The listing builds one solid part. Answer for the finished solid, in the listing's coordinates (mm). Give positions to 0.01 mm unless a question says otherwise; leave off trailing zeros. Write each loop counter-clockwise with the first axis right and the second up, starting at its lowest first coordinate (ties: lowest second). Pieces come first, ordered by that corner, then holes. Notation, with made-up numbers: M -10,25.5 L 18,25.5 A29 cw 18,58.5 Z; hole C -31,-17 d1. An arc over 180 degrees is marked long. Return JSON: item names as keys, results as strings.
from build123d import *

# Parameters (mm, degrees)
F2_DEPTH = 28.4
F3_DEPTH = 4
F6_D     = 5
F6_DEPTH = 5
F6_TIP   = 1.5021515476
F7_D     = 5
F7_DEPTH = 7
F7_TIP   = 1.5021515476
F8_R     = 1
F9_R     = 1.4485281374


with BuildPart() as f2:
    # F0 (on Front) → F2 (new body)
    with BuildSketch(Plane.XZ):
        with BuildLine():
            Line((23.6029717884, 8.2401288069), (37.7647548615, 13.1842060911))
            ThreePointArc((37.7647548615, 13.1842060911), (30.9779974122, 25.3054080451), (20.4548362885, 34.3744043208))
            Line((20.4548362885, 34.3744043208), (12.7842726803, 21.4840027005))
            ThreePointArc((12.7842726803, 21.4840027005), (19.3612483826, 15.8158800282), (23.6029717884, 8.2401288069))
        make_face()
    extrude(amount=F2_DEPTH)

    # F1 (on Front) + F0 (on Front) → F3 (join)
    with BuildSketch(Plane.XZ):
        with BuildLine():
            ThreePointArc((15.2340019476, 15.8721512297), (17.0378985767, 13.9179744248), (18.5928148308, 11.7604097152))
            Line((18.5928148308, 11.7604097152), (21.4911474241, 12.7722583124))
            ThreePointArc((21.4911474241, 12.7722583124), (22.6606475272, 10.5591218219), (23.6029717884, 8.2401288069))
            Line((23.6029717884, 8.2401288069), (37.7647548615, 13.1842060911))
            ThreePointArc((37.7647548615, 13.1842060911), (30.9779974122, 25.3054080451), (20.4548362885, 34.3744043208))
            Line((20.4548362885, 34.3744043208), (12.7842726803, 21.4840027005))
            ThreePointArc((12.7842726803, 21.4840027005), (14.8685909795, 20.0978855177), (16.8038497839, 18.5102845046))
            Line((16.8038497839, 18.5102845046), (15.2340019476, 15.8721512297))
        make_face()
    with BuildSketch(Plane.XZ):
        with BuildLine():
            Line((23.6029717884, 8.2401288069), (37.7647548615, 13.1842060911))
            ThreePointArc((37.7647548615, 13.1842060911), (30.9779974122, 25.3054080451), (20.4548362885, 34.3744043208))
            Line((20.4548362885, 34.3744043208), (12.7842726803, 21.4840027005))
            ThreePointArc((12.7842726803, 21.4840027005), (19.3612483826, 15.8158800282), (23.6029717884, 8.2401288069))
        make_face()
    extrude(amount=-F3_DEPTH)

    # F6 (one way)
    with BuildSketch(Plane(origin=(29.109795575, 0, 23.7793052059), x_dir=(0, 1, 0), z_dir=(-0.7744499353, 0, -0.6326352011))):
        with Locations((-5, 0)):
            Circle(F6_D / 2)
    extrude(amount=-F6_DEPTH, mode=Mode.SUBTRACT)
    with Locations(Plane(origin=(29.109795575, 0, 23.7793052059), x_dir=(0, 1, 0), z_dir=(-0.7744499353, 0, -0.6326352011))):
        with Locations((-5, 0)):
            with Locations((0, 0, -(F6_DEPTH + F6_TIP / 2))):  # 118° drill point
                Cone(0, F6_D / 2, F6_TIP, mode=Mode.SUBTRACT)

    # F7
    with Locations(Plane(origin=(29.109795575, 0, 23.7793052059), x_dir=(0, 1, 0), z_dir=(0.7744499353, 0, 0.6326352011))):
        with Locations((-5, 0)):
            Hole(F7_D / 2, depth=F7_DEPTH)
            with Locations((0, 0, -(F7_DEPTH + F7_TIP / 2))):  # 118° drill point
                Cone(0, F7_D / 2, F7_TIP, mode=Mode.SUBTRACT)

    # F8
    f8_edges = [f2.edges().sort_by_distance(p)[0] for p in [
        (21.491147, 2, 12.772258),
        (16.80385, 2, 18.510285),
    ]]
    fillet(f8_edges, radius=F8_R)

    # F9
    f9_edges = [f2.edges().sort_by_distance(p)[0] for p in [
        (17.037899, 4, 13.917974),
        (16.505655, 4, 18.471804),
        (21.393938, 4, 12.487739),
    ]]
    fillet(f9_edges, radius=F9_R)


solid = f2.part
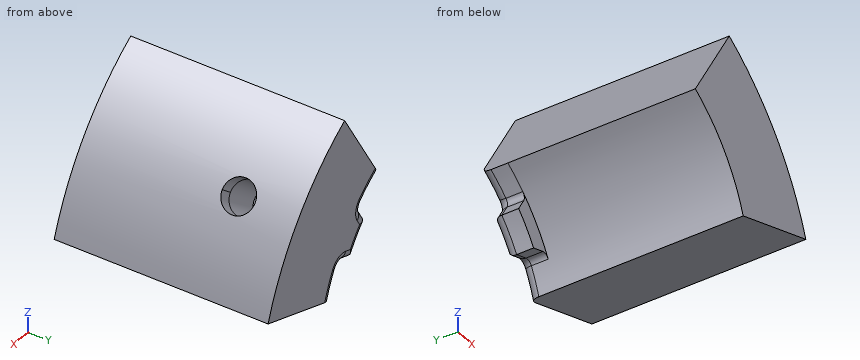
Item 1: Given pin 1 Ø8 at (y, z) = (-23.5, 27.5) entering from -X; pin 2 Ø6 at (x, y) = (34, -16.5) entering from -Z; pin 3 Ø10 at (y, z) = (-12, 15.5) entering from +X, each flat-ended and moving along its own axis, determine where each tip first touches the part or whether it passes through.
Geometry results:
{"pin 1": "stops at x = 13.98", "pin 2": "stops at z = 10.82", "pin 3": "stops at x = 37.76"}
Item 2: A cutting plane is placed at A-A, the plane y = -8.5. Write down the section's boundary in (x, z), plus the area to 3 significant figures.
Geometry results:
{"outline": "M 12.78,21.48 A25 cw 23.6,8.24 L 37.76,13.18 A40 ccw 20.45,34.37 Z", "area": "340 mm2"}
Item 3: Find the intervals of material crossed by line 1 (X direction, y = -1, z = 31.25); line 2 (Z direction, x = 23, y = -4.5); line 3 (X direction, y = -7, z = 20.5), in increasing order.
Geometry results:
{"line 1": "x = 18.6 to 24.97", "line 2": "z = 9.8 to 18.38, 21.95 to 32.73", "line 3": "x = 14.31 to 22.74, 27.47 to 34.35"}
Item 4: A cutting plane is placed at B-B, the plane x = 33.75. Write down the section's boundary in (y, z), plus the area to 3 significant figures.
Geometry results:
{"outline": "M -28.4,11.78 L 4,11.78 L 4,21.47 L -28.4,21.47 Z", "area": "314 mm2"}
